```python
from build123d import *

# Parameters (mm, degrees)
SKETCH1_W           = 13.5
SKETCH1_H           = 13.5
BOSS_EXTRUDE1_DEPTH = 19.7
SKETCH3_R           = 2
BOSS_EXTRUDE2_DEPTH = 12
SKETCH4_R           = 2
BOSS_EXTRUDE3_DEPTH = 12
FILLET1_R           = 0.5


with BuildPart() as part:
    # Sketch1 → Boss-Extrude1 (new body)
    with BuildSketch(Plane.XY):
        Rectangle(SKETCH1_W, SKETCH1_H)
    extrude(amount=BOSS_EXTRUDE1_DEPTH)

    # Sketch2 → Cut-Revolve1 (revolve, cut)
    with BuildSketch(Plane(origin=(0, 0, 0), x_dir=(1, 0, 0), z_dir=(0, 1, 0)), mode=Mode.PRIVATE) as cut_revolve1_sk:
        Polygon((-6.5, 0), (-15.39, 0), (-15.39, -19.7), (-6.5, -19.7), (-12.85, -16.033825791), (-12.85, -3.666174209), align=None)
    revolve(cut_revolve1_sk.sketch.rotate(Axis((0, 0, 20.715268644), (0, 0, -1)), 180), axis=Axis((0, 0, 20.715268644), (0, 0, -1)), mode=Mode.SUBTRACT)

    # Sketch3 → Boss-Extrude2 (add, symmetric)
    with BuildSketch(Plane(origin=(0, 0, 0), x_dir=(1, 0, 0), z_dir=(0, 1, 0))):
        with Locations(Location((0, -9.85, 0), (0, 0, 90))):
            Circle(SKETCH3_R)
    extrude(amount=BOSS_EXTRUDE2_DEPTH, both=True)

    # Sketch4 → Boss-Extrude3 (add, symmetric)
    with BuildSketch(Plane(origin=(0, 0, 0), x_dir=(0, 0, -1), z_dir=(1, 0, 0))):
        with Locations(Location((-9.85, 0, 0), (0, 0, 270))):
            Circle(SKETCH4_R)
    extrude(amount=BOSS_EXTRUDE3_DEPTH, both=True)

    # Fillet1
    fillet1_edges = [part.edges().sort_by_distance(p)[0] for p in [
        (0, -12, 11.85),
        (0, 12, 11.85),
        (-12, 2, 9.85),
        (12, 2, 9.85),
    ]]
    fillet(fillet1_edges, radius=FILLET1_R)


solid = part.part
```
Can you work these out from the model? Positions are in its coordinate system, mm. A direction names the side the tool comes from. Give positions to 0.01 mm unless a question says otherwise; leave off trailing zeros. Order: outer loops, then holes, each group sorted by start corner. A loop starts at its lowest first (then second) coordinate and runs counter-clockwise, first axis right, second up. Notation, with made-up numbers: M -33,53.25 L -2,53.25 A35 cw -2,89.25 Z; hole C -39.5,-14 d6. An arc over 180 degrees is marked long. One line per item, written item: value.
1) I want a section at A-A, the plane z = 9.85. List the corners of the cut face in (x, y) for me, plus the area to 3 significant figures.
Answer sheet:
outline: M -12,-1.5 A0.5 ccw -11.5,-2 L -6.75,-2 L -6.75,-6.75 L -2,-6.75 L -2,-11.5 A0.5 ccw -1.5,-12 L 1.5,-12 A0.5 ccw 2,-11.5 L 2,-6.75 L 6.75,-6.75 L 6.75,-2 L 11.5,-2 A0.5 ccw 12,-1.5 L 12,1.5 A0.5 ccw 11.5,2 L 6.75,2 L 6.75,6.75 L 2,6.75 L 2,11.5 A0.5 ccw 1.5,12 L -1.5,12 A0.5 ccw -2,11.5 L -2,6.75 L -6.75,6.75 L -6.75,2 L -11.5,2 A0.5 ccw -12,1.5 Z
area: 266 mm^2
2) I want a section at B-B, the plane x = 0. List the corners of the cut face in (y, z) for me, plus the area to 3 significant figures.
Answer sheet:
outline: M -12,8.35 A0.5 ccw -11.5,7.85 L -6.75,7.85 L -6.75,0.14 L -6.5,0 L 6.5,0 L 6.75,0.14 L 6.75,7.85 L 11.5,7.85 A0.5 ccw 12,8.35 L 12,11.35 A0.5 ccw 11.5,11.85 L 6.75,11.85 L 6.75,19.56 L 6.5,19.7 L -6.5,19.7 L -6.75,19.56 L -6.75,11.85 L -11.5,11.85 A0.5 ccw -12,11.35 Z
area: 308 mm^2
3) Please list where these lines run through material, in increasing order: line 1 along X through (y, z) = (6.25, 3); line 2 along Y through (x, z) = (-9.5, 10).
Answer sheet:
line 1: x = -6.75 to 6.75
line 2: y = -1.99 to 1.99
4) I want a section at D-D, the plane z = 12.5. List the corners of the cut face in (x, y) for me, plus the area to 3 significant figures.
Answer sheet:
outline: M -6.75,-6.75 L 6.75,-6.75 L 6.75,6.75 L -6.75,6.75 Z
area: 182 mm^2
5) For P1, Ø1.5, axis at x = -4, z = 11.5, coming from the +Y side; P2, Ø1, axis at x = -6, z = 7.5, coming from the -Y side; P3, Ø2, axis at y = 5.5, z = 4, coming from the +X side, each with a flat end and sliding along its axis, tell me the tip position at first contact or that it passes through.
Answer sheet:
P1: stops at y = 6.75
P2: stops at y = -6.75
P3: stops at x = 6.75
6) On a 3-axis mill with a long thin cutter (end or side, diameter ignored), from which of +Z, -Z, +X, -X, +Y, -Y can I reach the whole of each face in a straight line? I mean faces 1 (the face through (-9.092, 0.434, 11.802)), 2 (the face through (0.766, 9.158, 8.003)), 3 (the face through (9.158, 0.434, 11.802)), 4 (the face through (0.766, -9.092, 8.003)). Say none if no direction works.
Answer sheet:
face 1: -X
face 2: +Y
face 3: +X
face 4: -Y
